Part model, mm, in its own coordinate system. Face numbers are marked on the shaded views. Round coordinates to 2 decimals unless told otherwise and drop trailing zeros. Order: outer loops, then holes, each group sorted by start corner. A loop starts at its lowest first (then second) coordinate and runs counter-clockwise, first axis right, second up. Notation, with made-up numbers: (-12.5, 58) -> (5.5, 58) arc R12 ccw to (5.5, 75) -> close; hole circle Ø6 at (77, 37.25). An arc over 180 degrees is marked (long way). Answer as a JSON object with one key per item and string values. Group by question number.
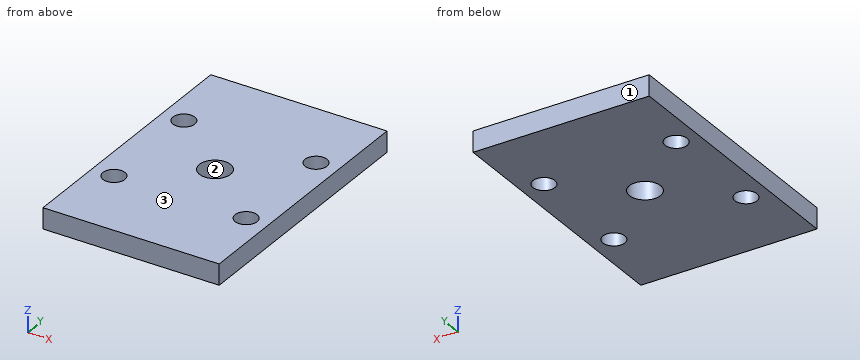
```python
from build123d import *

# Parameters (mm, degrees)
SKETCH1_W                   = 50.8
SKETCH1_H                   = 76.2
BOSS_EXTRUDE1_DEPTH         = 6
F_1_4_0_25_DIAMETER_HOLE1_D = 6.35
SKETCH5_R                   = 4.5
CUT_EXTRUDE1_DEPTH          = 7


with BuildPart() as part:
    # Sketch1 → Boss-Extrude1 (new body)
    with BuildSketch(Plane.XY):
        with Locations((25.4, 38.1)):
            Rectangle(SKETCH1_W, SKETCH1_H)
    extrude(amount=BOSS_EXTRUDE1_DEPTH)

    # 1/4 (0.25) Diameter Hole1 (through all)
    with Locations(Plane.XY.offset(6)):
        with Locations((44.45, 53.975), (6.35, 53.975), (6.35, 22.225), (44.45, 22.225)):
            Hole(F_1_4_0_25_DIAMETER_HOLE1_D / 2)

    # Sketch5 → Cut-Extrude1 (cut, through all)
    with BuildSketch(Plane.XY.offset(6)):
        with Locations((25.4, 38.1)):
            Circle(SKETCH5_R)
    extrude(amount=-CUT_EXTRUDE1_DEPTH, mode=Mode.SUBTRACT)


solid = part.part
```
Q1. Band-saw the part on A-A (x = 25.4). List the corners of the cut face in (y, z), plus the area to 3 significant figures.
Q2. Two-plate mould, pull along Y, no slides. Class the marked faces 1, 2 and 3: +Y half, -Y half, draft (parallel to the pull), parting line (faces both ways), or undercut.
Q3. Drop a flat-ended pin along its axis: pin 1 Ø5 at (x, y) = (44.45, 53.975) entering from +Z. Give the stop position or say it passes through.
Q4. Band-saw the part on B-B (y = 38.1). List the corners of the cut face in (x, z).
Q5. Band-saw the part on C-C (x = 6.35). List the corners of the cut face in (y, z), plus the area to 3 significant figures.
Q6. Wall check: line 1 (Y direction, x = 44.45, z = 3.55); line 2 (Y direction, x = 25.5, z = 4.1); line 3 (Y direction, x = 43, z = 1.4). Give the ranges that are in metal, low to high. Write a range as [from, to].
Q7. Band-saw the part on D-D (y = 56). List the corners of the cut face in (x, z), plus the area to 3 significant figures.
Completed:
{
 "1": {"outline": "(0, 0) -> (33.6, 0) -> (33.6, 6) -> (0, 6) -> close; (42.6, 0) -> (76.2, 0) -> (76.2, 6) -> (42.6, 6) -> close", "area": "403 mm2"},
 "2": {"face 1": "+Y half", "face 2": "undercut", "face 3": "draft"},
 "3": {"pin 1": "through"},
 "4": {"outline": "(0, 0) -> (20.9, 0) -> (20.9, 6) -> (0, 6) -> close; (29.9, 0) -> (50.8, 0) -> (50.8, 6) -> (29.9, 6) -> close"},
 "5": {"outline": "(0, 0) -> (19.05, 0) -> (19.05, 6) -> (0, 6) -> close; (25.4, 0) -> (50.8, 0) -> (50.8, 6) -> (25.4, 6) -> close; (57.15, 0) -> (76.2, 0) -> (76.2, 6) -> (57.15, 6) -> close", "area": "381 mm2"},
 "6": {"line 1": "[0, 19.05], [25.4, 50.8], [57.15, 76.2]", "line 2": "[0, 33.6], [42.6, 76.2]", "line 3": "[0, 19.4], [25.05, 51.15], [56.8, 76.2]"},
 "7": {"outline": "(0, 0) -> (3.9, 0) -> (3.9, 6) -> (0, 6) -> close; (8.8, 0) -> (42, 0) -> (42, 6) -> (8.8, 6) -> close; (46.9, 0) -> (50.8, 0) -> (50.8, 6) -> (46.9, 6) -> close", "area": "246 mm2"}
}
